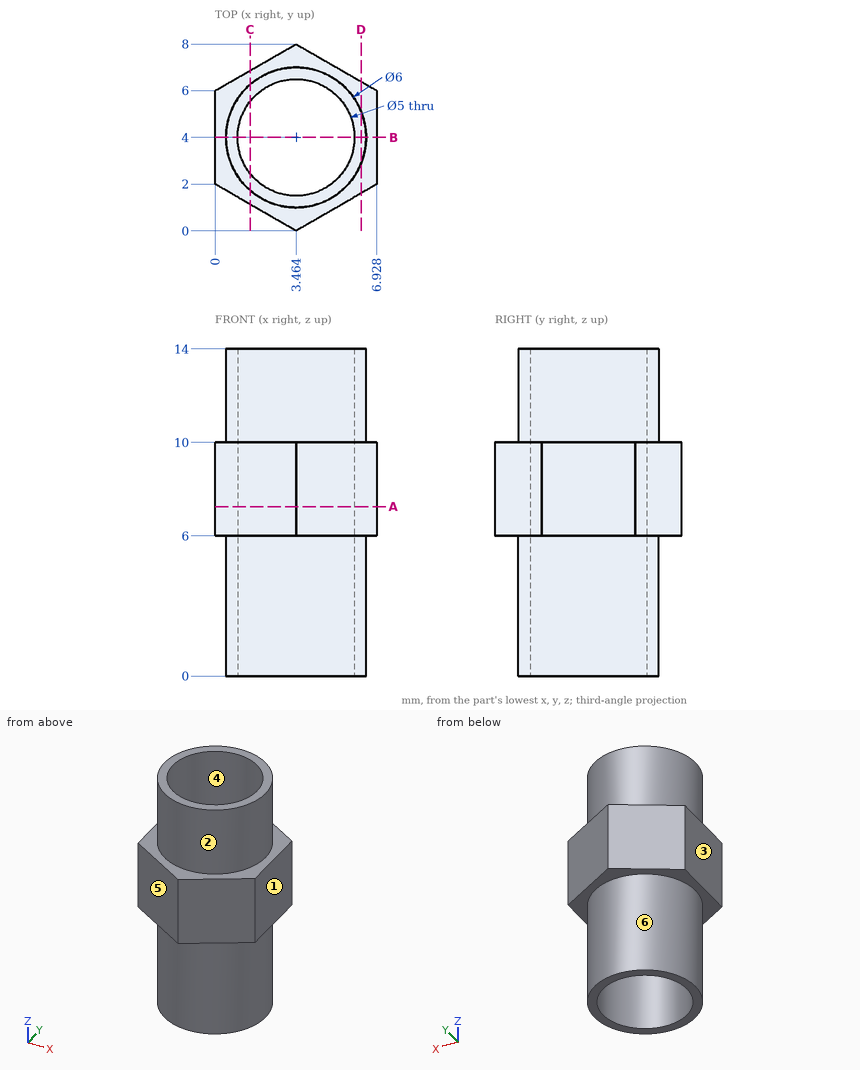
Input: dimensioned drawing with shaded views. Units: mm. Origin: part minimum x, y, z. A direction names the side the tool comes from. Round coordinates to 2 decimals unless told otherwise and drop trailing zeros. Loops run counter-clockwise (first coordinate to the right, second up) from the corner with the lowest first, then second, coordinate; pieces in that order, holes last.
1) Section query A-A on z = 7.25. Return the cut outline in (x, y).
Ans:
outline: (0, 2) - (3.46, 0) - (6.93, 2) - (6.93, 6) - (3.46, 8) - (0, 6) - close; hole circle Ø5 at (3.46, 4)
2) Pull-direction query (X, two-part tool) for the marked faces 1, 2, 3 and 4; classes: released by +X, released by -X, zero draft, split by the parting line, or undercut.
Ans:
face 1: released by +X
face 2: split by the parting line
face 3: released by -X
face 4: undercut
3) Section query C-C on x = 1.5. Return the cut outline in (y, z).
Ans:
outline: (1.13, 6) - (1.73, 6) - (1.73, 0) - (2.45, 0) - (2.45, 14) - (1.73, 14) - (1.73, 10) - (1.13, 10) - close; (5.55, 0) - (6.27, 0) - (6.27, 6) - (6.87, 6) - (6.87, 10) - (6.27, 10) - (6.27, 14) - (5.55, 14) - close
4) Pin query (flat end, axial travel): pin 1 (2 mm diameter, centred on x = 4, y = 5, fed in from -Z); pin 2 (1.5 mm diameter, centred on x = 3.5, z = 11, fed in from +Y). Return the tip coordinate at first contact, or that it passes through.
Ans:
pin 1: passes through
pin 2: stops at y = 7
5) Material intervals for line 1 (X direction, y = 4, z = 9.75); line 2 (Y direction, x = 3.5, z = 2.25); line 3 (X direction, y = 5.5, z = 7) (1 decimal), sorted ascending.
Ans:
line 1: x = 0 to 0.96, 5.96 to 6.93
line 2: y = 1 to 1.5, 6.5 to 7
line 3: x = 0 to 1.5, 5.5 to 6.9
6) Set-up query: the marked faces 5 and 6. Return all of +Z, -Z, +X, -X, +Y, -Y with unobstructed straight access to the full face (end or side cutting, diameter ignored); none if empty.
Ans:
face 5: +Z, -Z, -X, -Y
face 6: -Z
7) Section query D-D on x = 6.25. Return the cut outline in (y, z), plus the area to 3 significant figures.
Ans:
outline: (1.61, 6) - (2.89, 6) - (2.89, 0) - (5.11, 0) - (5.11, 6) - (6.39, 6) - (6.39, 10) - (5.11, 10) - (5.11, 14) - (2.89, 14) - (2.89, 10) - (1.61, 10) - close
area: 41.4 mm2
8) Section query B-B on y = 4. Return the cut outline in (x, z).
Ans:
outline: (0, 6) - (0.46, 6) - (0.46, 0) - (0.96, 0) - (0.96, 14) - (0.46, 14) - (0.46, 10) - (0, 10) - close; (5.96, 0) - (6.46, 0) - (6.46, 6) - (6.93, 6) - (6.93, 10) - (6.46, 10) - (6.46, 14) - (5.96, 14) - close
